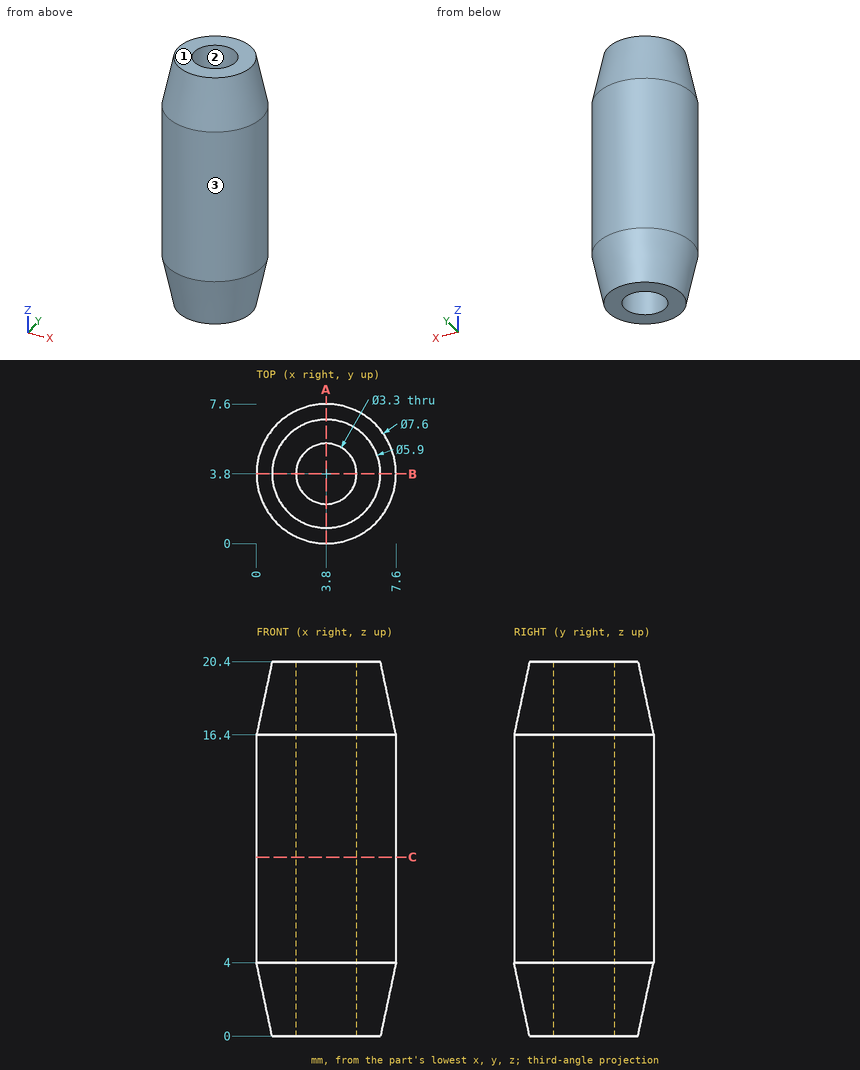
Print and shaded views of the part. All mm, measured from the part's lowest x, y and z. Give positions to 0.01 mm unless a question says otherwise; leave off trailing zeros. Loops run counter-clockwise (first coordinate to the right, second up) from the corner with the lowest first, then second, coordinate; pieces in that order, holes last.
1) Wall check: line 1 (Y direction, x = 3.8, z = 8.75); line 2 (Y direction, x = 4.75, z = 11.75); line 3 (X direction, y = 4.25, z = 17.5). Give the ranges that are in metal, low to high.
2) Pull direction X, two halves, no side cores. Call the marked faces 1, 2 and 3: +X half, -X half, draft (parallel to the pull), parting line (faces both ways), or undercut.
3) Saw through at C-C (z = 9.75). Write the cut outline in (x, y), plus the area to 3 significant figures.
4) Flat gauge pins, fed straight in: pin 1 Ø2 at (x, y) = (3.8, 3.8) entering from +Z (3 decimals); pin 2 Ø4 at (y, z) = (6, 3.5) entering from +X; pin 3 Ø1.5 at (x, z) = (6, 7) entering from +Y; pin 4 Ø3 at (y, z) = (6.5, 9.5) entering from -X (1 decimal). Where does each tip first touch, or does it go through?
5) Saw through at A-A (x = 3.8). Write the cut outline in (y, z).
Answer block:
1. line 1: y = 0 to 2.15, 5.45 to 7.6
1. line 2: y = 0.12 to 2.45, 5.15 to 7.48
1. line 3: x = 0.26 to 2.21, 5.39 to 7.34
2. face 1: draft
2. face 2: undercut
2. face 3: parting line
3. outline: circle Ø7.6 at (3.8, 3.8); hole circle Ø3.3 at (3.8, 3.8)
3. area: 36.8 mm2
4. pin 1: passes through
4. pin 2: stops at x = 7.59
4. pin 3: stops at y = 7.31
4. pin 4: stops at x = 0.2
5. outline: (0, 4) - (0.85, 0) - (2.15, 0) - (2.15, 20.4) - (0.85, 20.4) - (0, 16.4) - close; (5.45, 0) - (6.75, 0) - (7.6, 4) - (7.6, 16.4) - (6.75, 20.4) - (5.45, 20.4) - close
